For this review, take the finished solid that the model builds, in its own axes (mm). A direction names the side the tool comes from. Give positions to 0.01 mm unless a question says otherwise; leave off trailing zeros. Answer as a JSON object with one key per item and string values. Group by question number.
from build123d import *

# Parameters (mm, degrees)
SKETCH1_R                       = 5.3975
BOSS_EXTRUDE1_DEPTH             = 71.12
SKETCH8_R                       = 1.3208
CUT_EXTRUDE1_DEPTH              = 72.12
SKETCH10_R                      = 5.3975
SKETCH10_R_2                    = 4.7625
CUT_EXTRUDE2_DEPTH              = 12.7
F_1_4_0_25_DIAMETER_HOLE1_D     = 6.35
F_1_4_0_25_DIAMETER_HOLE1_DEPTH = 60.96
F_1_4_0_25_DIAMETER_HOLE1_TIP   = 1.907732465
CHAMFER1_SIZE2                  = 0.635
CHAMFER1_SIZE                   = 0.782829938


with BuildPart() as part:
    # Sketch1 → Boss-Extrude1 (new body)
    with BuildSketch(Plane.XY):
        Circle(SKETCH1_R)
    extrude(amount=BOSS_EXTRUDE1_DEPTH)

    # Sketch7 → Cut-Revolve1 (revolve, cut)
    with BuildSketch(Plane(origin=(0, 0, 0), x_dir=(1, 0, 0), z_dir=(0, 1, 0))):
        Polygon((5.3975, -71.12), (5.3975, -53.113680223), (2.2225, -71.12), align=None)
    revolve(axis=Axis((0, 0, -47.573976859), (0, 0, 1)), mode=Mode.SUBTRACT)

    # Sketch8 → Cut-Extrude1 (cut, through all)
    with BuildSketch(Plane.XY.offset(71.12)):
        Circle(SKETCH8_R)
    extrude(amount=-CUT_EXTRUDE1_DEPTH, mode=Mode.SUBTRACT)

    # Sketch10 → Cut-Extrude2 (cut)
    with BuildSketch(Plane(origin=(0, 0, 0), x_dir=(-1, 0, 0), z_dir=(0, 0, -1))):
        Circle(SKETCH10_R)
        Circle(SKETCH10_R_2, mode=Mode.SUBTRACT)
    extrude(amount=-CUT_EXTRUDE2_DEPTH, mode=Mode.SUBTRACT)

    # 1/4 (0.25) Diameter Hole1
    with Locations(Plane(origin=(0, 0, 0), x_dir=(-1, 0, 0), z_dir=(0, 0, -1))):
        with Locations((0, 0)):
            Hole(F_1_4_0_25_DIAMETER_HOLE1_D / 2, depth=F_1_4_0_25_DIAMETER_HOLE1_DEPTH)
            with Locations((0, 0, -(F_1_4_0_25_DIAMETER_HOLE1_DEPTH + F_1_4_0_25_DIAMETER_HOLE1_TIP / 2))):  # 118° drill point
                Cone(0, F_1_4_0_25_DIAMETER_HOLE1_D / 2, F_1_4_0_25_DIAMETER_HOLE1_TIP, mode=Mode.SUBTRACT)

    # Sketch18 → Cut-Revolve2 (revolve, cut)
    with BuildSketch(Plane(origin=(0, 0, 0), x_dir=(1, 0, 0), z_dir=(0, 1, 0))):
        with BuildLine():
            Line((4.7625, -12.7), (4.1656, -12.7))
            ThreePointArc((4.1656, -12.7), (3.6576, -12.192), (4.1656, -11.684))
            Line((4.1656, -11.684), (4.7625, -11.684))
            Line((4.7625, -11.684), (4.7625, -12.7))
        make_face()
    revolve(axis=Axis((0, 0, 0.466216552), (0, 0, -1)), mode=Mode.SUBTRACT)

    # Sketch20 → Cut-Revolve3 (revolve, cut)
    with BuildSketch(Plane(origin=(0, 0, 0), x_dir=(1, 0, 0), z_dir=(0, 1, 0))):
        Polygon((4.7625, 0), (4.7625, -1.2319), (3.5306, 0), align=None)
    revolve(axis=Axis((0, 0, 0.466216552), (0, 0, -1)), mode=Mode.SUBTRACT)

    # Chamfer1
    chamfer1_edges = [part.edges().sort_by_distance(p)[0] for p in [
        (-2.2225, 0, 71.12),
    ]]
    chamfer(chamfer1_edges, length=CHAMFER1_SIZE, length2=CHAMFER1_SIZE2)


solid = part.part
1) For faces 1 (the face through (-0.69, -3.1, 30.91)), 2 (the face through (-3.853, 0.17, 61.852)), 3 (the face through (-2, 4, 11.684)), list the 3-axis set-ups (+Z, -Z, +X, -X, +Y, -Y) from which the entire face can be reached by the end or side of a thin tool; tool diameter is ignored.
2) Mouldability with a two-part tool opening along Y and no side actions: class faces 4 (the face through (-1.05, -0.8, 66.66)), 5 (the face through (-3.978, 3.648, 32.624)), 6 (the face through (-2, -4, 12.7)) as released by +Y, released by -Y, zero draft, split by the parting line, or undercut.
3) For line 1 (Y direction, x = -0.25, z = 33); line 2 (X direction, y = 1.75, z = 43.5); line 3 (X direction, y = 1.75, z = 56), list the stretches that pass through material, from the lowest coordinate up.
4) For pin 1 (1 mm diameter, centred on x = 4.5, z = 27, fed in from +Y); pin 2 (1.5 mm diameter, centred on y = 2, z = 30.5, fed in from -X); pin 3 (2 mm diameter, centred on x = 1, z = 55, fed in from -Y), all flat-tipped, find the tip position at first contact; note any pin that passes through.
Result set:
{
 "1": {"face 1": "-Z", "face 2": "+Z", "face 3": "none"},
 "2": {"face 4": "undercut", "face 5": "split by the parting line", "face 6": "zero draft"},
 "3": {"line 1": "y = -5.39 to -3.17, 3.17 to 5.39", "line 2": "x = -5.11 to -2.65, 2.65 to 5.11", "line 3": "x = -4.56 to -2.65, 2.65 to 4.56"},
 "4": {"pin 1": "stops at y = 3.62", "pin 2": "stops at x = -5.25", "pin 3": "stops at y = -5.19"}
}
